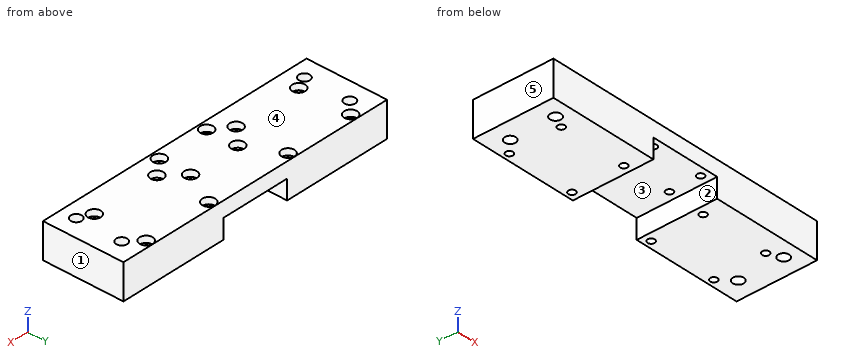
from build123d import *

# Parameters (mm, degrees)
BOSS_EXTRUDE1_DEPTH            = 31
M10X1_5_TAPPED_HOLE1_D         = 8.5
CBORE_FOR_M5_SHCS1_D           = 5.5
CBORE_FOR_M5_SHCS1_CBORE_D     = 10
CBORE_FOR_M5_SHCS1_CBORE_DEPTH = 5
CBORE_FOR_M5_SHCS2_D           = 5.5
CBORE_FOR_M5_SHCS2_CBORE_D     = 10
CBORE_FOR_M5_SHCS2_CBORE_DEPTH = 5


with BuildPart() as part:
    # Sketch1 → Boss-Extrude1 (new, symmetric)
    with BuildSketch(Plane(origin=(0, 0, 0), x_dir=(1, 0, 0), z_dir=(0, 1, 0))):
        Polygon((-27, 0), (27, 0), (27, 15.1), (111.5, 15.1), (111.5, -11.9), (-111.5, -11.9), (-111.5, 15.1), (-27, 15.1), align=None)
    extrude(amount=BOSS_EXTRUDE1_DEPTH, both=True)

    # M10x1.5 Tapped Hole1 (through all)
    with Locations(Plane.XY.offset(11.9)):
        with Locations((-96.5, 16), (-96.5, -19), (96.5, 16), (96.5, -19)):
            Hole(M10X1_5_TAPPED_HOLE1_D / 2)

    # CBORE for M5 SHCS1 (through all)
    with Locations(Plane.XY.offset(11.9)):
        with Locations((-86.5, 25.75), (-86.5, -14.25), (-33.5, 25.75), (-33.5, -14.25), (33.5, 25.75), (86.5, 25.75), (33.5, -14.25), (86.5, -14.25)):
            CounterBoreHole(CBORE_FOR_M5_SHCS1_D / 2, CBORE_FOR_M5_SHCS1_CBORE_D / 2, CBORE_FOR_M5_SHCS1_CBORE_DEPTH)

    # CBORE for M5 SHCS2 (through all)
    with Locations(Plane.XY.offset(11.9)):
        with Locations((-20, -0.65), (20, -0.65), (20, -24.65), (-20, -24.65)):
            CounterBoreHole(CBORE_FOR_M5_SHCS2_D / 2, CBORE_FOR_M5_SHCS2_CBORE_D / 2, CBORE_FOR_M5_SHCS2_CBORE_DEPTH)


solid = part.part
The listing builds one solid part. Answer for the finished solid, in the listing's coordinates (mm). Face numbers are marked on the shaded views. A direction names the side the tool comes from. Give positions to 0.01 mm unless a question says otherwise; leave off trailing zeros. Write each loop counter-clockwise with the first axis right and the second up, starting at its lowest first coordinate (ties: lowest second). Pieces come first, ordered by that corner, then holes. Notation, with made-up numbers: (85.25, 53) - (134.25, 53) arc R34 cw to (134.25, 92) - close; hole circle Ø11 at (31, 9.25). An arc over 180 degrees is marked (long way). Use a Markdown table: item, result.
1. For a pull along X with two mould halves and no side action, classify the marked faces 3, 4 and 5 as released by +X, released by -X, zero draft, split by the parting line, or undercut.
Values follow:
| item | result |
|---|---|
| face 3 | undercut |
| face 4 | zero draft |
| face 5 | released by -X |
2. Find the intervals of material crossed by probe 1 along Y at (x, z) = (20, 3); probe 2 along X at (y, z) = (-8, -1.75); probe 3 along X at (y, z) = (1, 9.75), in increasing order. Write a range as from..to.
Values follow:
| item | result |
|---|---|
| probe 1 | y = -31..-27.4, -21.9..-3.4, 2.1..31 |
| probe 2 | x = -111.5..-27, 27..111.5 |
| probe 3 | x = -111.5..-24.72, -15.28..15.28, 24.72..111.5 |
3. A tool of negligible diameter and unlimited length cuts with its end or side. For the marked faces 1 and 2, from which of +Z, -Z, +X, -X, +Y, -Y can it reach the whole face along a straight path? Write none if from no direction.
Values follow:
| item | result |
|---|---|
| face 1 | +Z, -Z, +X, +Y, -Y |
| face 2 | -Z, +Y, -Y |
4. Section C-C on x = -96.5 is taken. Write down the section's boundary in (y, z), plus the area to 4 significant figures.
Values follow:
| item | result |
|---|---|
| outline | (-31, -15.1) - (-23.25, -15.1) - (-23.25, 11.9) - (-31, 11.9) - close; (-14.75, -15.1) - (11.75, -15.1) - (11.75, 11.9) - (-14.75, 11.9) - close; (20.25, -15.1) - (31, -15.1) - (31, 11.9) - (20.25, 11.9) - close |
| area | 1,215 mm² |
5. Each of these flat-tipped pins is pushed along its axis until it touches: P1, Ø9, axis at x = 20, y = -0.65, coming from the +Z side; P2, Ø3.5, axis at x = -20, y = -0.65, coming from the -Z side; P3, Ø2, axis at x = -7, y = -22, coming from the -Z side. Where does it stop, or does it pass through?
Values follow:
| item | result |
|---|---|
| P1 | stops at z = 6.9 |
| P2 | passes through |
| P3 | stops at z = 0 |
6. Section A-A on z = -12.5 is taken. Count the separate pieces of the cut face and the enclosed holes in it, plus the area to 3 significant figures.
Values follow:
| item | result |
|---|---|
| separate pieces | 2 |
| enclosed holes | 12 |
| area | 10,100 mm² |
7. Section B-B on x = -20 is taken. Write down the section's boundary in (y, z).
Values follow:
| item | result |
|---|---|
| outline | (-31, 0) - (-27.4, 0) - (-27.4, 6.9) - (-29.65, 6.9) - (-29.65, 11.9) - (-31, 11.9) - close; (-21.9, 0) - (-3.4, 0) - (-3.4, 6.9) - (-5.65, 6.9) - (-5.65, 11.9) - (-19.65, 11.9) - (-19.65, 6.9) - (-21.9, 6.9) - close; (2.1, 0) - (31, 0) - (31, 11.9) - (4.35, 11.9) - (4.35, 6.9) - (2.1, 6.9) - close |
